For this review, take the finished solid that the model builds, in its own axes (mm). Coordinates: 2 decimals unless noted, no trailing zeros. Loops run counter-clockwise (first coordinate to the right, second up) from the corner with the lowest first, then second, coordinate; pieces in that order, holes last. Notation, with made-up numbers: M 48,-29 L 62,-29 A15 cw 62,-10 Z; hole C 44,70 d11. An arc over 180 degrees is marked long. Put each result on its own line as item: value.
```python
from build123d import *

# Parameters (mm, degrees)
SKETCH_W             = 107
SKETCH_H             = 72
PAD_DEPTH            = 2
SKETCH001_W          = 1
SKETCH001_H          = 64
PAD001_DEPTH         = 3
SKETCH002_W          = 1
SKETCH002_H          = 64
PAD002_DEPTH         = 2
SKETCH003_W          = 1
SKETCH003_H          = 64
PAD003_DEPTH         = 2
SKETCH004_W          = 1
SKETCH004_H          = 64
PAD004_DEPTH         = 3
SKETCH005_W          = 99
SKETCH005_H          = 1
PAD005_DEPTH         = 3
SKETCH006_W          = 99
SKETCH006_H          = 1
PAD006_DEPTH         = 2
SKETCH007_W          = 99
SKETCH007_H          = 1
PAD007_DEPTH         = 2
SKETCH008_W          = 99
SKETCH008_H          = 1
PAD008_DEPTH         = 3
SKETCH009_W          = 102
SKETCH009_H          = 15
POCKET_DEPTH         = 3.001
POCKET_DEPTH_BACK    = 2.001
SKETCH010_W          = 99.896225
SKETCH010_H          = 50
POCKET001_DEPTH      = 2.001
SKETCH011_W          = 10
SKETCH011_H          = 72
PAD009_DEPTH         = 2
SKETCH012_R          = 2.25
POCKET002_DEPTH      = 2.001
SKETCH014_W          = 10
SKETCH014_H          = 72
PAD010_DEPTH         = 2
SKETCH013_R          = 2.25
POCKET003_DEPTH      = 2.001
SKETCH015_W          = 102
SKETCH015_H          = 15
POCKET004_DEPTH      = 2
POCKET004_DEPTH_BACK = 2


with BuildPart() as part:
    # Sketch → Pad (new body)
    with BuildSketch(Plane.XY):
        with Locations((53.5, 36)):
            Rectangle(SKETCH_W, SKETCH_H)
    extrude(amount=-PAD_DEPTH)

    # Sketch001 → Pad001 (join)
    with BuildSketch(Plane.XY):
        with Locations((0.5, 36)):
            Rectangle(SKETCH001_W, SKETCH001_H)
    extrude(amount=PAD001_DEPTH)

    # Sketch002 → Pad002 (join)
    with BuildSketch(Plane.XY):
        with Locations((3, 36)):
            Rectangle(SKETCH002_W, SKETCH002_H)
    extrude(amount=PAD002_DEPTH)

    # Sketch003 → Pad003 (join)
    with BuildSketch(Plane.XY):
        with Locations((104, 36)):
            Rectangle(SKETCH003_W, SKETCH003_H)
    extrude(amount=PAD003_DEPTH)

    # Sketch004 → Pad004 (join)
    with BuildSketch(Plane.XY):
        with Locations((106.5, 36)):
            Rectangle(SKETCH004_W, SKETCH004_H)
    extrude(amount=PAD004_DEPTH)

    # Sketch005 → Pad005 (join)
    with BuildSketch(Plane.XY):
        with Locations((53.5, 71.5)):
            Rectangle(SKETCH005_W, SKETCH005_H)
    extrude(amount=PAD005_DEPTH)

    # Sketch006 → Pad006 (join)
    with BuildSketch(Plane.XY):
        with Locations((53.5, 69)):
            Rectangle(SKETCH006_W, SKETCH006_H)
    extrude(amount=PAD006_DEPTH)

    # Sketch007 → Pad007 (join)
    with BuildSketch(Plane.XY):
        with Locations((53.5, 3)):
            Rectangle(SKETCH007_W, SKETCH007_H)
    extrude(amount=PAD007_DEPTH)

    # Sketch008 → Pad008 (join)
    with BuildSketch(Plane.XY):
        with Locations((53.5, 0.5)):
            Rectangle(SKETCH008_W, SKETCH008_H)
    extrude(amount=PAD008_DEPTH)

    # Sketch009 → Pocket (cut, two sides)
    with BuildSketch(Plane.XY) as pocket_sk:
        with Locations((53.5, 11.2)):
            Rectangle(SKETCH009_W, SKETCH009_H)
    extrude(amount=POCKET_DEPTH, mode=Mode.SUBTRACT)
    extrude(pocket_sk.sketch, amount=-POCKET_DEPTH_BACK, mode=Mode.SUBTRACT)

    # Sketch010 → Pocket001 (cut, through all)
    with BuildSketch(Plane.XY):
        with Locations((53.448113, 43.5)):
            Rectangle(SKETCH010_W, SKETCH010_H)
    extrude(amount=-POCKET001_DEPTH, mode=Mode.SUBTRACT)

    # Sketch011 → Pad009 (join)
    with BuildSketch(Plane.XY):
        with Locations((-5, 36)):
            Rectangle(SKETCH011_W, SKETCH011_H)
    extrude(amount=-PAD009_DEPTH)

    # Sketch012 → Pocket002 (cut, through all)
    with BuildSketch(Plane.XY):
        with Locations((-5, 5)):
            Circle(SKETCH012_R)
        with Locations((-5, 36)):
            Circle(SKETCH012_R)
        with Locations((-5, 67)):
            Circle(SKETCH012_R)
    extrude(amount=-POCKET002_DEPTH, mode=Mode.SUBTRACT)

    # Sketch014 → Pad010 (join)
    with BuildSketch(Plane.XY):
        with Locations((112, 36)):
            Rectangle(SKETCH014_W, SKETCH014_H)
    extrude(amount=-PAD010_DEPTH)

    # Sketch013 → Pocket003 (cut, through all)
    with BuildSketch(Plane.XY):
        with Locations((112, 5)):
            Circle(SKETCH013_R)
        with Locations((112, 36)):
            Circle(SKETCH013_R)
        with Locations((112, 67)):
            Circle(SKETCH013_R)
    extrude(amount=-POCKET003_DEPTH, mode=Mode.SUBTRACT)

    # Sketch015 → Pocket004 (cut, two sides)
    with BuildSketch(Plane.XY) as pocket004_sk:
        with Locations((53.5, 60.6)):
            Rectangle(SKETCH015_W, SKETCH015_H)
    extrude(amount=POCKET004_DEPTH, mode=Mode.SUBTRACT)
    extrude(pocket004_sk.sketch, amount=-POCKET004_DEPTH_BACK, mode=Mode.SUBTRACT)


solid = part.part
```
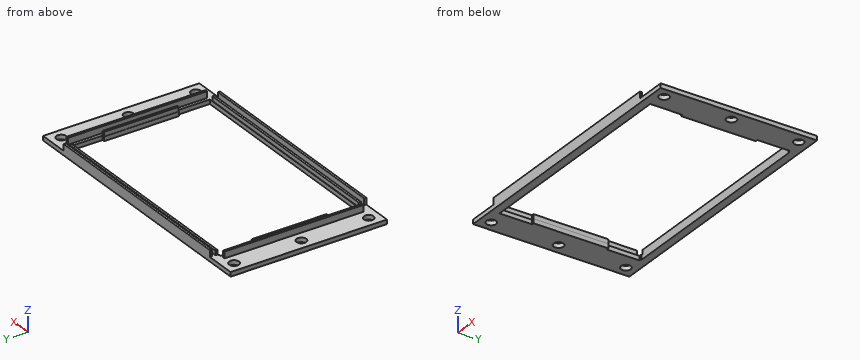
(1) Add section B-B (y = 9.5). Write out the cut boundary in (x, z), plus the area to 3 significant figures.
Determined:
outline: M -10,-2 L 2.5,-2 L 2.5,0 L 1,0 L 1,3 L 0,3 L 0,0 L -10,0 Z; M 104.5,-2 L 117,-2 L 117,0 L 107,0 L 107,3 L 106,3 L 106,0 L 104.5,0 Z
area: 56.0 mm^2
(2) For pin 1 (2 mm diameter, centred on y = 20, z = 1.5, fed in from +X); pin 2 (5 mm diameter, centred on x = 112, y = 67, fed in from +Z); pin 3 (1.1 mm diameter, centred on x = 106.5, z = 1, fed in from +Y), all flat-tipped, find the tip position at first contact; note any pin that passes through.
Determined:
pin 1: stops at x = 107
pin 2: stops at z = 0
pin 3: stops at y = 68
(3) Wall thickness on line 1 along Y through (x, z) = (-5, -0.95); line 2 along X through (y, z) = (25, 1.1); line 3 along Y through (x, z) = (15.5, 1.45): over which ranges is each line inside the solid? List them lowest first. Write a range as [from, to].
Determined:
line 1: y = [0, 2.75], [7.25, 33.75], [38.25, 64.75], [69.25, 72]
line 2: x = [0, 1], [2.5, 3.5], [103.5, 104.5], [106, 107]
line 3: y = [0, 1], [2.5, 3.5], [68.5, 69.5], [71, 72]
(4) Add section A-A (x = 112). Write out the cut boundary in (y, z).
Determined:
outline: M 0,-2 L 2.75,-2 L 2.75,0 L 0,0 Z; M 7.25,-2 L 33.75,-2 L 33.75,0 L 7.25,0 Z; M 38.25,-2 L 64.75,-2 L 64.75,0 L 38.25,0 Z; M 69.25,-2 L 72,-2 L 72,0 L 69.25,0 Z
(5) Add section C-C (z = 0.8). State how many separate pieces and enclosed holes the cut face has, plus the area to 3 significant figures.
Determined:
separate pieces: 8
enclosed holes: 0
area: 593 mm^2
